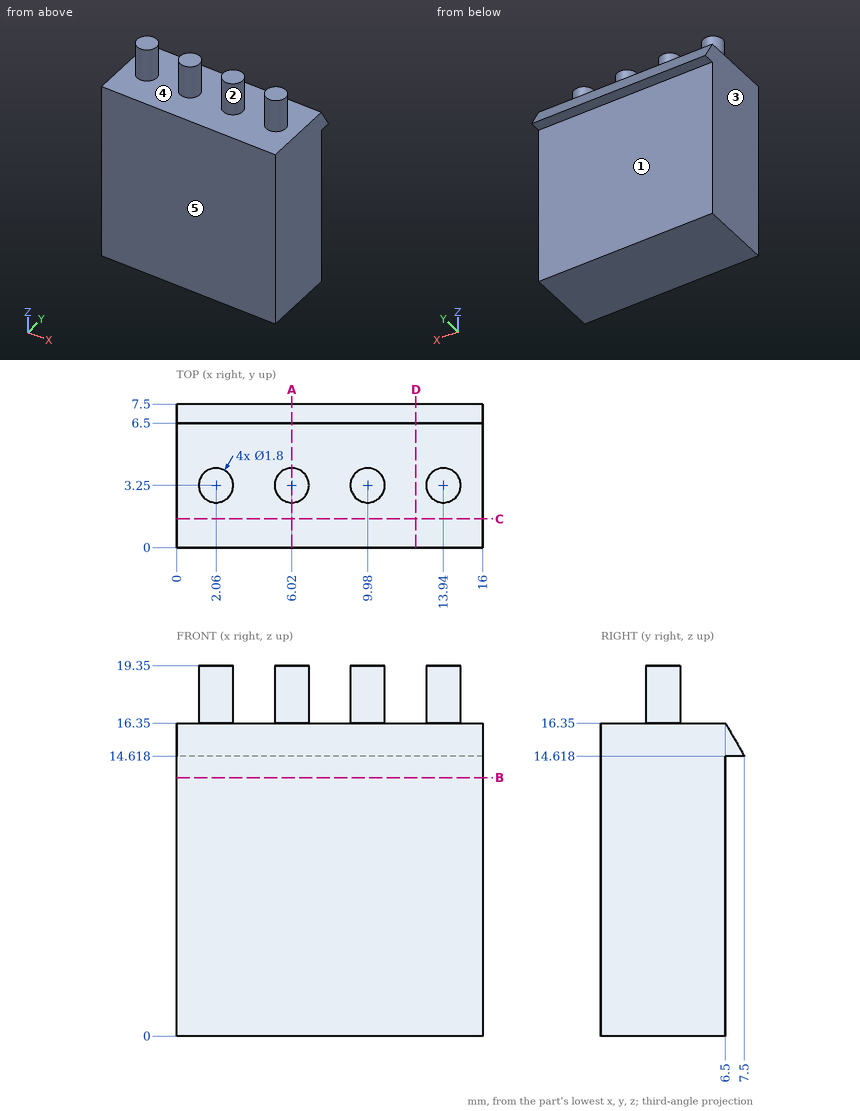
Design review of the part shown in the three views and the two pictorial views. Dimensions are in mm from the part's minimum x, y and z. A direction names the side the tool comes from. Coordinates: 2 decimals unless noted, no trailing zeros. Write each loop counter-clockwise with the first axis right and the second up, starting at its lowest first coordinate (ties: lowest second). Pieces come first, ordered by that corner, then holes.
1) We need section A-A on x = 6.02. State the section outline as (y, z) points, then the cut area to 3 significant figures.
2) Clearance check with flat-ended pins moving along their axes: pin 1 Ø0.8 at (x, y) = (6.5, 7) entering from -Z; pin 2 Ø6 at (x, z) = (5.5, 10) entering from +Y. State where each tip first meets the part, or that it passes through.
3) We need section C-C on y = 1.5. State the section outline as (x, z) points.
4) We need section D-D on x = 12.5. State the section outline as (y, z) points.
5) The part is to be moulded in two halves that separate along X. For the marked faces 1, 2 and 3, say which applies: pulls with the +X half, pulls with the -X half, needs draft (parallel to the pull), parting line crosses it, or undercut.
6) To check wall thickness, follow probe 1 along Z at (x, y) = (6.75, 6.25); probe 2 along Y at (x, z) = (11, 1); probe 3 along Z at (x, y) = (4.75, 7.25). State the ranges of each line that lie inside material, in increasing order.
7) Machinability: for the marked faces 4 and 5, which of the approach directions +Z, -Z, +X, -X, +Y, -Y give a long, thin tool a straight path to every point of the face, cutting with its end or side? Answer none if there is none.
8) We need section B-B on z = 13.5. State the section outline as (x, y) points, then the cut area to 3 significant figures.
Answer list:
1. outline: (0, 0) - (6.5, 0) - (6.5, 14.62) - (7.5, 14.62) - (6.5, 16.35) - (4.15, 16.35) - (4.15, 19.35) - (2.35, 19.35) - (2.35, 16.35) - (0, 16.35) - close
1. area: 113 mm2
2. pin 1: stops at z = 14.62
2. pin 2: stops at y = 6.5
3. outline: (0, 0) - (16, 0) - (16, 16.35) - (0, 16.35) - close
4. outline: (0, 0) - (6.5, 0) - (6.5, 14.62) - (7.5, 14.62) - (6.5, 16.35) - (0, 16.35) - close
5. face 1: needs draft
5. face 2: undercut
5. face 3: pulls with the -X half
6. probe 1: z = 0 to 16.35
6. probe 2: y = 0 to 6.5
6. probe 3: z = 14.62 to 15.05
7. face 4: +Z
7. face 5: +Z, -Z, +X, -X, -Y
8. outline: (0, 0) - (16, 0) - (16, 6.5) - (0, 6.5) - close
8. area: 104 mm2
